from build123d import *

# Parameters (mm, degrees)
F1_DEPTH = 63.5
F0_W     = 25.4
F0_H     = 19.05
F2_DEPTH = 25.4
F3_DEPTH = 9.2075
F5_R     = 6.35
F6_R     = 11.3954507036
F7_DEPTH = 76.201


with BuildPart() as f1:
    # F0 (on Front) → F1 (new body, symmetric)
    with BuildSketch(Plane.XZ):
        Polygon((-41.275, 9.525), (-41.275, -9.525), (41.275, -9.525), (41.275, 9.525), (22.225, 9.525), align=None)
    extrude(amount=F1_DEPTH, both=True)

    # F0 (on Front) → F2 (join, symmetric)
    with BuildSketch(Plane.XZ):
        with BuildLine():
            Line((22.225, 9.525), (41.275, 9.525))
            Line((41.275, 9.525), (41.275, 27.0002))
            ThreePointArc((41.275, 27.0002), (45.9246798487, 38.2255201513), (57.15, 42.8752))
            Line((57.15, 42.8752), (60.325, 42.8752))
            Line((60.325, 42.8752), (60.325, 61.9252))
            Line((60.325, 61.9252), (57.15, 61.9252))
            add(Edge.make_bspline(
                [(53.2009990256, 61.7012232746), (54.5754497046, 61.8116519501), (55.8942153415, 61.886670259), (57.15, 61.9252)],
                knots=[106.938445779, 106.938445779, 106.938445779, 106.938445779, 111.5045361635, 111.5045361635, 111.5045361635, 111.5045361635], degree=3))
            ThreePointArc((53.2009990256, 61.7012232746), (31.0954947847, 50.2578521383), (22.225, 27.0002))
            Line((22.225, 27.0002), (22.225, 9.525))
        make_face()
        with Locations((73.025, 52.4002)):
            Rectangle(F0_W, F0_H)
    extrude(amount=F2_DEPTH, both=True)

    # F0 (on Front) → F3 (join, symmetric)
    with BuildSketch(Plane.XZ):
        with BuildLine():
            add(Edge.make_bspline(
                [(-41.275, 9.525), (-41.7220303949, 37.1060348211), (21.011180815, 59.1149689658), (53.2009990256, 61.7012232746)],
                knots=[0, 0, 0, 0, 106.938445779, 106.938445779, 106.938445779, 106.938445779], degree=3))
            Line((-41.275, 9.525), (22.225, 9.525))
            Line((22.225, 9.525), (22.225, 27.0002))
            ThreePointArc((22.225, 27.0002), (31.0954947847, 50.2578521383), (53.2009990256, 61.7012232746))
        make_face()
    extrude(amount=F3_DEPTH, both=True)

    # F0 (on Front) → F4 (revolve)
    with BuildSketch(Plane.XZ):
        Polygon((85.725, 66.675), (85.725, 61.9252), (85.725, 42.8752), (85.725, 38.1), (111.125, 38.1), (111.125, 66.675), align=None)
    revolve(axis=Axis((85.725, 0, 52.3875), (0, 0, 1)))

    # F5
    f5_edges = [f1.edges().sort_by_distance(p)[0] for p in [
        (41.275, -63.5, 0),
        (-41.275, -63.5, 0),
        (-41.275, 63.5, 0),
        (41.275, 63.5, 0),
    ]]
    fillet(f5_edges, radius=F5_R)

    # F6 (on face) → F7 (cut, through all)
    with BuildSketch(Plane.XY.offset(66.675)):
        with Locations((85.725, 0)):
            Circle(F6_R)
    extrude(amount=-F7_DEPTH, mode=Mode.SUBTRACT)


solid = f1.part
Verification items for the finished model (mm, model axes). A direction names the side the tool comes from. Coordinates: 2 decimals unless noted, no trailing zeros. Order: outer loops, then holes, each group sorted by start corner. A loop starts at its lowest first (then second) coordinate and runs counter-clockwise, first axis right, second up. Notation, with made-up numbers: M -23.5,42.5 L -12.5,42.5 A18 ccw -12.5,49.5 Z; hole C 17,79.5 d11. An arc over 180 degrees is marked long. One line per item, written item: value. Start each with the question number.
Item 1: Thickness scan on probe 1 along Z at (x, y) = (-7, 48) (3 decimals); probe 2 along Y at (x, z) = (-23, 32); probe 3 along Y at (x, z) = (45, 47). Record the ranges inside material, lowest first.
Item 2: Access from +Z, -Z, +X, -X, +Y, -Y to the whole of each face (thin tool, end or side, straight path). Record for faces 4 (the flat face through (41.275, -1, 4)), 5 (the cylindrical face through (31.33, 17.19, 50.52)), 6 (the flat face through (46, -25.4, 42)), 7 (the flat face through (22.225, -17, 18)), 8 (the flat face through (60, -2, 61.925)).
Item 3: Sectioned sample at A-A on y = 39.5. Record the cut outline in (x, z) (3 decimals), then the cut area to 3 significant figures.
Item 4: Sectioned sample at B-B on x = 62.5. Record the cut outline in (y, z) (3 decimals), then the cut area to 3 significant figures.
Item 5: Depth check by flat-ended pin: P1, Ø15.5, axis at x = 60, z = 42, coming from the +Y side; P2, Ø6, axis at x = 83, z = 39.5, coming from the -Y side; P3, Ø6, axis at y = -21, z = 46.5, coming from the -X side. Enter the tip coordinate at first touch or a pass-through.
Item 6: Mould release check, pull along Y, two halves, no side actions. Record for faces 1 (the cylindrical face through (96.6, 3.4, 52.6)), 2 (the flat face through (46, 25.4, 42)), 3 (the flat face through (22.225, 17, 18)): pulls with the +Y half, pulls with the -Y half, needs draft (parallel to the pull), parting line crosses it, or undercut.
Calculated:
1. probe 1: -9.525 to 9.525
1. probe 2: -9.21 to 9.21
1. probe 3: -25.4 to 25.4
2. face 4: -Z, +X, +Y, -Y
2. face 5: +Z, -X, +Y
2. face 6: +Z, +X, -X, -Y
2. face 7: +Z, -X, -Y
2. face 8: +Z, -X
3. outline: M -41.275,-9.525 L 41.275,-9.525 L 41.275,9.525 L -41.275,9.525 Z
3. area: 1,570 mm^2
4. outline: M -25.4,42.875 L -10.284,42.875 L -10.284,38.1 L 10.284,38.1 L 10.284,42.875 L 25.4,42.875 L 25.4,61.925 L 10.284,61.925 L 10.284,66.675 L -10.284,66.675 L -10.284,61.925 L -25.4,61.925 Z
4. area: 1,160 mm^2
5. P1: y = 25.4
5. P2: y = -25.4
5. P3: x = 26.37
6. face 1: undercut
6. face 2: pulls with the +Y half
6. face 3: needs draft
